```python
from build123d import *

# Parameters (mm, degrees)
SKETCH_1_R        = 9.4
SKETCH_1_R_2      = 7.4
EXTRUDE_1_DEPTH   = 4.9
SKETCH_2_W        = 5.498524857
SKETCH_2_H        = 3.9
EXTRUDE_1_2_DEPTH = 3.9


with BuildPart() as part:
    # 草图1 → Extrude 1 (new body)
    with BuildSketch(Plane.XY):
        Circle(SKETCH_1_R)
        Circle(SKETCH_1_R_2, mode=Mode.SUBTRACT)
    extrude(amount=EXTRUDE_1_DEPTH)

    # 草图2 → Extrude 1 2 (add)
    with BuildSketch(Plane.XY):
        with Locations((5.39294726, 0)):
            Rectangle(SKETCH_2_W, SKETCH_2_H)
        with Locations((-5.39294726, 0)):
            Rectangle(SKETCH_2_W, SKETCH_2_H)
    extrude(amount=EXTRUDE_1_2_DEPTH)


solid = part.part
```
Geometry: final body of the model. Coordinates: model frame, mm. A direction names the side the tool comes from. Round coordinates to 2 decimals unless told otherwise and drop trailing zeros. Write each loop counter-clockwise with the first axis right and the second up, starting at its lowest first coordinate (ties: lowest second). Pieces come first, ordered by that corner, then holes. Notation, with made-up numbers: (83.5, -37) -> (113.5, -37) arc R17 ccw to (113.5, -19) -> close; hole circle Ø11 at (-27, 78.5). An arc over 180 degrees is marked (long way). Return JSON: item names as keys, results as strings.
Q1. Set-up query: faces 4 (the flat face through (-5, 0, 3.9)), 5 (the flat face through (3, -7, 4.9)), 6 (the flat face through (2.644, 0, 2)). Return all of +Z, -Z, +X, -X, +Y, -Y with unobstructed straight access to the full face (end or side cutting, diameter ignored); none if empty.
From the geometry:
{"face 4": "+Z", "face 5": "+Z, +X, -X, +Y, -Y", "face 6": "+Z, -Z"}
Q2. Section A-A on y = 0. Return the cut outline in (x, z).
From the geometry:
{"outline": "(-9.4, 0) -> (-2.64, 0) -> (-2.64, 3.9) -> (-7.4, 3.9) -> (-7.4, 4.9) -> (-9.4, 4.9) -> close; (2.64, 0) -> (9.4, 0) -> (9.4, 4.9) -> (7.4, 4.9) -> (7.4, 3.9) -> (2.64, 3.9) -> close"}
Q3. Ray query, line 1 (Y direction, x = 0, z = 1.5); line 2 (Y direction, x = -4.5, z = 0.55); line 3 (X direction, y = 0.75, z = 4.2). Return the intervals inside material, ascending.
From the geometry:
{"line 1": "-9.4 to -7.4, 7.4 to 9.4", "line 2": "-8.25 to -5.87, -1.95 to 1.95, 5.87 to 8.25", "line 3": "-9.37 to -7.36, 7.36 to 9.37"}
Q4. First-contact query: pin 1 Ø2 at (y, z) = (-6, 3) entering from +X; pin 2 Ø1.2 at (x, z) = (-4.5, 2.5) entering from -Y; pin 3 Ø1.5 at (y, z) = (-4.5, 3) entering from -X. Flat tips, straight axial feed; report the tip coordinate or a pass-through.
From the geometry:
{"pin 1": "x = 7.96", "pin 2": "y = -8.55", "pin 3": "x = -8.62"}
Q5. Section B-B on x = 0. Return the cut outline in (y, z), and give its area (3 significant figures).
From the geometry:
{"outline": "(-9.4, 0) -> (-7.4, 0) -> (-7.4, 4.9) -> (-9.4, 4.9) -> close; (7.4, 0) -> (9.4, 0) -> (9.4, 4.9) -> (7.4, 4.9) -> close", "area": "19.6 mm2"}
Q6. Section C-C on z = 2.1. Return the cut outline in (x, y), and give its area (3 significant figures).
From the geometry:
{"outline": "circle Ø18.8 at (0, 0); hole (-7.14, -1.95) arc R7.4 ccw to (7.14, -1.95) -> (2.64, -1.95) -> (2.64, 1.95) -> (7.14, 1.95) arc R7.4 ccw to (-7.14, 1.95) -> (-2.64, 1.95) -> (-2.64, -1.95) -> close", "area": "142 mm2"}
Q7. Section D-D on x = -6.5. Return the cut outline in (y, z), and give its area (3 significant figures).
From the geometry:
{"outline": "(-6.79, 0) -> (-3.54, 0) -> (-3.54, 4.9) -> (-6.79, 4.9) -> close; (-1.95, 0) -> (1.95, 0) -> (1.95, 3.9) -> (-1.95, 3.9) -> close; (3.54, 0) -> (6.79, 0) -> (6.79, 4.9) -> (3.54, 4.9) -> close", "area": "47.1 mm2"}
Q8. Mould query, pull axis Y, two halves, no side actions, for faces 1 (the flat face through (5, 0, 3.9)), 2 (the cylindrical face through (-2.038, -9.176, 2.416)), 3 (the flat face through (4, 0, 0)). Classes: +Y half, -Y half, draft (parallel to the pull), parting line (faces both ways), or undercut.
From the geometry:
{"face 1": "undercut", "face 2": "parting line", "face 3": "draft"}
